Build history of the part. All positions in model axes, mm. Give positions to 0.01 mm unless a question says otherwise; leave off trailing zeros. Write each loop counter-clockwise with the first axis right and the second up, starting at its lowest first coordinate (ties: lowest second). Pieces come first, ordered by that corner, then holes. Notation, with made-up numbers: (4, 29) - (9, 29) arc R21 ccw to (9, 34) - close; hole circle Ø9 at (-33.75, 71.5). An arc over 180 degrees is marked (long way). Use one line per item in the form item = value. Start each with the question number.
from build123d import *

# Parameters (mm, degrees)
F2_DEPTH = 900
F3_R     = 4.25
F4_DEPTH = 1.2000000005


with BuildPart() as f2:
    # F0 (on Top) → F2 (new body)
    with BuildSketch(Plane.XY):
        with BuildLine():
            ThreePointArc((12.5006749989, 22.499625), (11.7684949852, 24.2674139192), (10.00075, 24.9996999989))
            Line((10.00075, 24.9997), (-9.99925, 25.000299))
            ThreePointArc((-9.99925, 25.0002989989), (-11.7670389192, 24.2681189852), (-12.4993249989, 22.500374))
            Line((-12.499325, 22.500374), (-12.49955, 15.000374))
            Line((-12.49955, 15.000374), (-11.29955, 15.000338))
            Line((-11.29955, 15.000338), (-11.299325, 22.500338))
            ThreePointArc((-11.2993249994, 22.500338), (-10.918536238, 23.4195653923), (-9.999286, 23.8002989994))
            Line((-9.999286, 23.800299), (10.000714, 23.7997))
            ThreePointArc((10.000714, 23.7996999994), (10.9199413923, 23.418911238), (11.3006749994, 22.499661))
            Line((11.300675, 22.499661), (11.299326, -22.500339))
            ThreePointArc((11.2993259994, -22.500339), (10.918537238, -23.4195663923), (9.999287, -23.8002999994))
            Line((9.999287, -23.8003), (-10.000713, -23.799701))
            ThreePointArc((-10.000713, -23.7997009994), (-10.9199403923, -23.418912238), (-11.3006739994, -22.499662))
            Line((-11.300674, -22.499662), (-11.30045, -14.999662))
            Line((-11.30045, -14.999662), (-12.50045, -14.999626))
            Line((-12.50045, -14.999626), (-12.500674, -22.499626))
            ThreePointArc((-12.5006739989, -22.499626), (-11.7684939852, -24.2674149192), (-10.000749, -24.9997009989))
            Line((-10.000749, -24.999701), (9.999251, -25.0003))
            ThreePointArc((9.999251, -25.0002999989), (11.7670399192, -24.2681199852), (12.4993259989, -22.500375))
            Line((12.499326, -22.500375), (12.500675, 22.499625))
        make_face()
    extrude(amount=F2_DEPTH)

    # F3 (on face) → F4 (cut, through all)
    with BuildSketch(Plane(origin=(12.5000005, -0.0003747222, 0), x_dir=(2.99778e-05, 0.9999999996, 0), z_dir=(0.9999999996, -2.99778e-05, 0))):
        with Locations((0, 22)):
            Circle(F3_R)
        with Locations((0, 878)):
            Circle(F3_R)
    extrude(amount=-F4_DEPTH, mode=Mode.SUBTRACT)


solid = f2.part
(1) Pin check, flat tips, straight feed: pin 1 Ø11 at (y, z) = (0, 22) entering from -X; pin 2 Ø7 at (y, z) = (0, 878) entering from +X; pin 3 Ø8 at (x, y) = (9, -10) entering from -Z. Stop position of each tip, or through.
(2) Wall check: line 1 (Y direction, x = -7.75, z = 355); line 2 (X direction, y = 17.5, z = 845.5); line 3 (X direction, y = 7, z = 153). Give the ranges that are in metal, low to high. Write a range as from..to.
(3) Cut at B-B, the plane z = 176. Give the cut face in (x, y), then the cut area to 3 significant figures.
(4) Cut at A-A, the plane x = 1.25. Give the cut face in (y, z), then the cut area to 3 significant figures.
Solution:
q1.pin_1 = 11.3
q1.pin_2 = through
q1.pin_3 = 0
q2.line_1 = -25..-23.8, 23.8..25
q2.line_2 = -12.5..-11.3, 11.3..12.5
q2.line_3 = 11.3..12.5
q3.outline = (-12.5, -22.5) arc R2.5 ccw to (-10, -25) - (10, -25) arc R2.5 ccw to (12.5, -22.5) - (12.5, 22.5) arc R2.5 ccw to (10, 25) - (-10, 25) arc R2.5 ccw to (-12.5, 22.5) - (-12.5, 15) - (-11.3, 15) - (-11.3, 22.5) arc R1.3 cw to (-10, 23.8) - (10, 23.8) arc R1.3 cw to (11.3, 22.5) - (11.3, -22.5) arc R1.3 cw to (10, -23.8) - (-10, -23.8) arc R1.3 cw to (-11.3, -22.5) - (-11.3, -15) - (-12.5, -15) - close
q3.area = 134 mm2
q4.outline = (-25, 0) - (-23.8, 0) - (-23.8, 900) - (-25, 900) - close; (23.8, 0) - (25, 0) - (25, 900) - (23.8, 900) - close
q4.area = 2,160 mm2
